```python
from build123d import *

# Parameters (mm, degrees)
F2_R     = 6
F3_DEPTH = 1.5
F5_DEPTH = 9.5
F6_D     = 3.3
F6_DEPTH = 4.5
F6_TIP   = 0.9914200214


with BuildPart() as f1:
    # F0 (on Front) → F1 (revolve)
    with BuildSketch(Plane.XZ):
        Polygon((-78.9, 16.1), (-78.9, 0), (0, 0), (0, 17.7), (-33.6, 17.7), (-33.6, 16.1), align=None)
    revolve(axis=Axis((-39.45, 0, 0), (-1, 0, 0)))

    # F2 (on face) → F3 (join)
    with BuildSketch(Plane.YZ):
        with Locations((0, 8.73)):
            Circle(F2_R)
    extrude(amount=F3_DEPTH)

    # F4 (on face) → F5 (join)
    with BuildSketch(Plane.YZ.offset(1.5)):
        with BuildLine():
            Line((2, 10.23), (-2, 10.23))
            ThreePointArc((-2, 10.23), (0, 6.23), (2, 10.23))
        make_face()
    extrude(amount=F5_DEPTH)

    # F6
    with Locations(Plane.YZ):
        with Locations((-10.25, 8.73), (10.25, 8.73), (0, -13.37)):
            Hole(F6_D / 2, depth=F6_DEPTH)
            with Locations((0, 0, -(F6_DEPTH + F6_TIP / 2))):  # 118° drill point
                Cone(0, F6_D / 2, F6_TIP, mode=Mode.SUBTRACT)


solid = f1.part
```
Build history of the part. All positions in model axes, mm. A direction names the side the tool comes from. Round coordinates to 2 decimals unless told otherwise and drop trailing zeros. Order: outer loops, then holes, each group sorted by start corner. A loop starts at its lowest first (then second) coordinate and runs counter-clockwise, first axis right, second up. Notation, with made-up numbers: (-4.5, -9.75) -> (3.5, -9.75) arc R19 ccw to (3.5, 3.25) -> close; hole circle Ø7 at (62, 62.5). An arc over 180 degrees is marked (long way). Answer in a Markdown table with one row per item.
1) Band-saw the part on A-A on z = 0. Give the cut face in (x, y).
Values:
| item | result |
|---|---|
| outline | (-78.9, -16.1) -> (-33.6, -16.1) -> (-33.6, -17.7) -> (0, -17.7) -> (0, 17.7) -> (-33.6, 17.7) -> (-33.6, 16.1) -> (-78.9, 16.1) -> close |
2) Which spindle directions (+Z, -Z, +X, -X, +Y, -Y) get a long thin tool onto all of the face, cutting with end or side? Do faces 1 (the cylindrical face through (-2.281, 8.676, 9.226)), 2 (the flat face through (6, 0, 10.23)), 3 (the flat face through (-33.6, -16, 4)). Say none if no direction does.
Values:
| item | result |
|---|---|
| face 1 | +X |
| face 2 | +Z, +X, +Y, -Y |
| face 3 | -X |
3) Band-saw the part on D-D on z = 12. Give the cut face in (x, y).
Values:
| item | result |
|---|---|
| outline | (-78.9, -10.73) -> (-33.6, -10.73) -> (-33.6, -13.01) -> (0, -13.01) -> (0, -5.03) -> (1.5, -5.03) -> (1.5, 5.03) -> (0, 5.03) -> (0, 13.01) -> (-33.6, 13.01) -> (-33.6, 10.73) -> (-78.9, 10.73) -> close |
4) Wall check: L1, parallel to Y at x = -1.9, z = 8.73; L2, parallel to X at y = 0.5, z = 12.5; L3, parallel to X at y = 4, z = -12. Give the ranges that are in metal, low to high.
Values:
| item | result |
|---|---|
| L1 | -15.4 to -11.9, -8.6 to 8.6, 11.9 to 15.4 |
| L2 | -78.9 to 1.5 |
| L3 | -78.9 to 0 |
5) Mould opens along Z. For faces 4 (the flat face through (-78.9, 0, 0)), 5 (the conical face through (-5.32, 10.51, 8.62)), 6 (the cylindrical face through (-56.567, 4.836, 15.357)) say: released by +Z, released by -Z, zero draft, split by the parting line, or undercut.
Values:
| item | result |
|---|---|
| face 4 | zero draft |
| face 5 | undercut |
| face 6 | split by the parting line |
6) Band-saw the part on C-C on x = -40. Give the cut face in (y, z).
Values:
| item | result |
|---|---|
| outline | circle Ø32.2 at (0, 0) |
7) Band-saw the part on B-B on y = 15. Give the cut face in (x, z), and give its area (3 significant figures).
Values:
| item | result |
|---|---|
| outline | (-78.9, -5.85) -> (-33.6, -5.85) -> (-33.6, -9.4) -> (0, -9.4) -> (0, 9.4) -> (-33.6, 9.4) -> (-33.6, 5.85) -> (-78.9, 5.85) -> close |
| area | 1,160 mm2 |
8) Pin check, flat tips, straight feed: P1, Ø2, axis at x = 5, y = 0, coming from the +Z side; P2, Ø1.5, axis at y = 1, z = 4.5, coming from the +X side; P3, Ø5, axis at x = -31.5, y = 8, coming from the -Z side. Stop position of each tip, or through.
Values:
| item | result |
|---|---|
| P1 | z = 10.23 |
| P2 | x = 1.5 |
| P3 | z = -16.82 |
